Geometry check sheet. Reference: the model listing, model coordinates, mm. A direction names the side the tool comes from. Give positions to 0.01 mm unless a question says otherwise; leave off trailing zeros. One line per question, with ' | ' between items.
from build123d import *

# Parameters (mm, degrees)
SKETCH1_W                 = 48.308864232
SKETCH1_H                 = 41.275
BOSS_EXTRUDE1_DEPTH       = 6.35
F_8_CLEARANCE_HOLE1_D     = 4.9149
F_1_4_CLEARANCE_HOLE1_D   = 7.14248
SKETCH9_W                 = 6.35
SKETCH9_H                 = 41.275
EXTRUDE_THIN1_DEPTH       = 8.255
CHAMFER2_SIZE             = 9.525
CUT_EXTRUDE1_DEPTH        = 156.127382276
CHAMFER1_SIZE             = 2.54
HOLE1_AT_2_COUNT          = 2
HOLE1_AT_2_PITCH          = 9.3599
F_2_CLEARANCE_HOLE1_D     = 2.7051
F_2_CLEARANCE_HOLE1_DEPTH = 3.175
CHAMFER3_SIZE             = 1.27


with BuildPart() as part:
    # Sketch1 → Boss-Extrude1 (new body)
    with BuildSketch(Plane.XY):
        with Locations((-124.004465969, -24.5875)):
            Rectangle(SKETCH1_W, SKETCH1_H)
    extrude(amount=BOSS_EXTRUDE1_DEPTH)

    # #8 Clearance Hole1 (through all)
    with Locations(Plane.XY.offset(6.35)):
        with Locations((-111.927249911, -24.5875), (-136.081682027, -24.5875)):
            Hole(F_8_CLEARANCE_HOLE1_D / 2)

    # 1/4 Clearance Hole1 (through all)
    with Locations(Plane.XY.offset(6.35)):
        with Locations((-124.004465969, -14.4275), (-124.004465969, -34.7475)):
            Hole(F_1_4_CLEARANCE_HOLE1_D / 2)

    # Sketch9 → Extrude-Thin1 (add)
    with BuildSketch(Plane.XY.offset(6.35)):
        with Locations((-103.025033853, -24.5875)):
            Rectangle(SKETCH9_W, SKETCH9_H)
        with Locations((-144.983898085, -24.5875)):
            Rectangle(SKETCH9_W, SKETCH9_H)
    extrude(amount=EXTRUDE_THIN1_DEPTH)

    # Chamfer2
    # the kernel refuses this chamfer: 9.525 mm, written as the material it adds along each edge
    with BuildSketch(Plane(origin=(-106.200033853, -3.95, 6.35), x_dir=(0.0274958766105871, 0, 0.9996219169112966), z_dir=(0, -1, 0))) as chamfer2_piece_1_section:
        Polygon((CHAMFER2_SIZE * 0.999621916911, CHAMFER2_SIZE * 0.0274958766106), (-CHAMFER2_SIZE * 0.0274958766106, CHAMFER2_SIZE * 0.999621916911), (0, 0), align=None)
    chamfer2_piece_1 = extrude(amount=41.275, mode=Mode.PRIVATE)
    chamfer2_piece_1 = chamfer2_piece_1 - Plane(origin=(-111.927249911, -24.5875, 9.368765613), x_dir=(-1, 0, 0), z_dir=(0, 0, -1)) * Cylinder(2.45745, 121, mode=Mode.PRIVATE)
    chamfer2_piece_1 = split(chamfer2_piece_1, bisect_by=Plane(origin=(-109.341812124, -24.58749874, 14.605), z_dir=(0, 0, -1)), keep=Keep.TOP, mode=Mode.PRIVATE)
    add(chamfer2_piece_1)
    with BuildSketch(Plane(origin=(-141.808898085, -45.225, 6.35), x_dir=(0.9996219169112968, 0, -0.027495876610586386), z_dir=(0, 1, 0))) as chamfer2_piece_2_section:
        Polygon((CHAMFER2_SIZE * 0.999621916911, -CHAMFER2_SIZE * 0.0274958766106), (-CHAMFER2_SIZE * 0.0274958766106, -CHAMFER2_SIZE * 0.999621916911), (0, 0), align=None)
    chamfer2_piece_2 = extrude(amount=41.275, mode=Mode.PRIVATE)
    chamfer2_piece_2 = chamfer2_piece_2 - Plane(origin=(-136.081682027, -24.5875, 9.368765819), x_dir=(-1, 0, 0), z_dir=(0, 0, -1)) * Cylinder(2.45745, 121, mode=Mode.PRIVATE)
    chamfer2_piece_2 = split(chamfer2_piece_2, bisect_by=Plane(origin=(-138.667118685, -24.587501904, 14.605), z_dir=(0, 0, -1)), keep=Keep.TOP, mode=Mode.PRIVATE)
    add(chamfer2_piece_2)

    # Sketch10 → Cut-Extrude1 (cut, through all)
    with BuildSketch(Plane.XY.offset(6.35)):
        with BuildLine():
            Line((-136.081682027, -18.2375), (-111.927249911, -18.2375))
            ThreePointArc((-111.927249911, -18.2375), (-105.577249911, -24.5875), (-111.927249911, -30.9375))
            Line((-111.927249911, -30.9375), (-136.081682027, -30.9375))
            ThreePointArc((-136.081682027, -30.9375), (-142.431682027, -24.5875), (-136.081682027, -18.2375))
        make_face()
    extrude(amount=CUT_EXTRUDE1_DEPTH, mode=Mode.SUBTRACT)

    # Chamfer1
    chamfer1_edges = [part.edges().sort_by_distance(p)[0] for p in [
        (-99.850033853, -45.225, 7.3025),
        (-148.158898085, -45.225, 7.3025),
        (-148.158898085, -3.95, 7.3025),
        (-99.850033853, -3.95, 7.3025),
    ]]
    chamfer(chamfer1_edges, length=CHAMFER1_SIZE)

    # Sketch12 → Hole1 (revolve, cut)
    with BuildSketch(Plane(origin=(-148.158898085, -26.4544, 7.4422), x_dir=(0, 0, 1), z_dir=(0, 1, 0))):
        Polygon((0, 0), (0, 2.921), (1.4986, 2.921), (1.6383, 0), align=None)
    hole1 = revolve(axis=Axis((-38.158898085, -26.4544, 7.4422), (-1, 0, 0)), mode=Mode.SUBTRACT)

    # Hole1 at 2: Hole1 ×2
    with Locations(*[(0, i * HOLE1_AT_2_PITCH, 0) for i in range(1, HOLE1_AT_2_COUNT)]):
        add(hole1, mode=Mode.SUBTRACT)

    # #2 Clearance Hole1
    with Locations(Plane.ZY.offset(148.158898085)):
        with Locations((7.4422, -17.0945), (7.4422, -26.4544)):
            Hole(F_2_CLEARANCE_HOLE1_D / 2, depth=F_2_CLEARANCE_HOLE1_DEPTH)

    # Chamfer3
    chamfer3_edges = [part.edges().sort_by_distance(p)[0] for p in [
        (-120.433225969, -34.7475, 0),
        (-120.433225969, -14.4275, 0),
    ]]
    chamfer(chamfer3_edges, length=CHAMFER3_SIZE)


solid = part.part
Item 1: Sectioned sample at B-B (z = 3). Give the number of separate pieces and of enclosed holes in the cut face, plus the area to 3 significant figures.
Result:
separate pieces: 1 | enclosed holes: 4 | area: 1,860 mm2
Item 2: Set-up check for faces 5 (the face through (-136.354, -37.28, 10.42)), 6 (the face through (-113, -30.938, 8)), 7 (the face through (-124, -45.225, 5)): record each of +Z, -Z, +X, -X, +Y, -Y from which the full face is reachable in a straight line by a thin tool's end or side.
Result:
face 5: +Z, +Y, -Y | face 6: +Z | face 7: +Z, -Z, +X, -X, -Y
Item 3: Scan lines: probe 1 along Y at (x, z) = (-124, 5.5) (3 decimals); probe 2 along Y at (x, z) = (-122, 5) (3 decimals); probe 3 along Z at (x, y) = (-128, -31). Record each from-to range of solid material in increasing order.
Result:
probe 1: -45.225 to -38.319, -31.176 to -17.999, -10.856 to -3.95 | probe 2: -45.225 to -37.703, -31.792 to -17.383, -11.472 to -3.95 | probe 3: 0 to 6.35
Item 4: Release check for a two-part mould opening along Y. For faces 1 (the face through (-146.719, -15.771, 8.286)), 2 (the face through (-127.41, -33.67, 3.77)), 3 (the face through (-101.102, -43.937, 7.2)), 4 (the face through (-136.354, -12.12, 10.42)) record: pulls with the +Y half, pulls with the -Y half, needs draft (parallel to the pull), parting line crosses it, or undercut.
Result:
face 1: undercut | face 2: undercut | face 3: pulls with the -Y half | face 4: needs draft
Item 5: Depth check by flat-ended pin: pin 1 Ø8 at (x, y) = (-124, -14.43) entering from -Z; pin 2 Ø6.5 at (x, y) = (-111.93, -24.59) entering from +Z; pin 3 Ø0.8 at (y, z) = (-26.5, 7.5) entering from -X. Enter the tip coordinate at first touch or a pass-through.
Result:
pin 1: z = 0.84 | pin 2: z = 6.35 | pin 3: x = -144.98
